from build123d import *

# Parameters (mm, degrees)
CROQUIS1_R              = 2.2
SALIENTE_EXTRUIR1_DEPTH = 8
CHAFL_N1_SIZE           = 3


with BuildPart() as part:
    # Croquis1 → Saliente-Extruir1 (new body)
    with BuildSketch(Plane.XY):
        with BuildLine():
            Line((-75, 0), (-60, 0))
            ThreePointArc((-60, 0), (0, 60), (60, 0))
            Line((60, 0), (75, 0))
            ThreePointArc((75, 0), (0, 75), (-75, 0))
        make_face()
        with Locations((0, 67.5)):
            Circle(CROQUIS1_R, mode=Mode.SUBTRACT)
        with Locations((-58.456714755, 33.75)):
            Circle(CROQUIS1_R, mode=Mode.SUBTRACT)
        with Locations((58.456714755, 33.75)):
            Circle(CROQUIS1_R, mode=Mode.SUBTRACT)
    extrude(amount=SALIENTE_EXTRUIR1_DEPTH)

    # Chaflán1
    chafl_n1_edges = [part.edges().sort_by_distance(p)[0] for p in [
        (0, 75, 8),
        (0, 60, 8),
    ]]
    chamfer(chafl_n1_edges, length=CHAFL_N1_SIZE)


solid = part.part
Here's how the part is built. I have some questions about the finished solid (model axes, mm). Give positions to 0.01 mm unless a question says otherwise; leave off trailing zeros. Order: outer loops, then holes, each group sorted by start corner. A loop starts at its lowest first (then second) coordinate and runs counter-clockwise, first axis right, second up. Notation, with made-up numbers: (7, -11) -> (13, -11) arc R28 ccw to (13, 27) -> close; hole circle Ø7 at (23, 58). An arc over 180 degrees is marked (long way). Use a Markdown table: item, result. Add a question column.
Item 1: Imagine slicing it at C-C on y = 33.75. Give the number of separate pieces and of enclosed holes in the cut face, plus the area to 3 significant figures.
Item 2: Will these pins go through, and if not, where does the flat tip stop? pin 1 (5.5 mm diameter, centred on x = -58.46, y = 33.75, fed in from -Z); pin 2 (1.5 mm diameter, centred on y = 16, z = 5.5, fed in from +X); pin 3 (1 mm diameter, centred on y = 38.5, z = 6.5, fed in from +X).
Item 3: Imagine slicing it at B-B on z = 6.5. Please give me the cut outline in (x, y), plus the area to 3 significant figures.
Item 4: If we mould it in two halves opening along Y, with no side actions, what happens to faces 1 (the face through (-1.319, 59.985, 2.465)), 2 (the face through (57.98, 31.602, 3.944)), 3 (the face through (5, 60, 0)), 4 (the face through (-60.2, 32.41, 3.94))? For each: pulls with the +Y half, pulls with the -Y half, needs draft (parallel to the pull), parting line crosses it, or undercut.
Item 5: Imagine slicing it at A-A on x = 0. Please give me the cut outline in (y, z).
Item 6: I need wall thicknesses on line 1 (Y direction, x = 0, z = 4); line 2 (X direction, y = 45, z = 6); line 3 (X direction, y = 15, z = 7.5). Which ranges of each line are inside material? Lowest first, please.
Data:
| question | item | result |
|---|---|---|
| 1 | separate pieces | 4 |
| 1 | enclosed holes | 0 |
| 1 | area | 187 mm² |
| 2 | pin 1 | stops at z = 0 |
| 2 | pin 2 | stops at x = 73.39 |
| 2 | pin 3 | stops at x = 63.27 |
| 3 | outline | (-73.5, 0) -> (-61.5, 0) arc R61.5 cw to (61.5, 0) -> (73.5, 0) arc R73.5 ccw to start; hole circle Ø4.4 at (-58.46, 33.75); hole circle Ø4.4 at (0, 67.5); hole circle Ø4.4 at (58.46, 33.75) |
| 3 | area | 2,500 mm² |
| 4 | face 1 | pulls with the -Y half |
| 4 | face 2 | undercut |
| 4 | face 3 | needs draft |
| 4 | face 4 | undercut |
| 5 | outline | (60, 0) -> (65.3, 0) -> (65.3, 8) -> (63, 8) -> (60, 5) -> close; (69.7, 0) -> (75, 0) -> (75, 5) -> (72, 8) -> (69.7, 8) -> close |
| 6 | line 1 | y = 60 to 65.3, 69.7 to 75 |
| 6 | line 2 | x = -58.75 to -41.18, 41.18 to 58.75 |
| 6 | line 3 | x = -70.93 to -60.67, 60.67 to 70.93 |
